from build123d import *

# Parameters (mm, degrees)
F3_DEPTH = 50
F2_R     = 25
F4_DEPTH = 15
F5_DEPTH = 35
F6_DEPTH = 35


with BuildPart() as f3:
    # F0 (on Front) → F3 (new body)
    with BuildSketch(Plane.XZ):
        with BuildLine():
            Line((0, 76), (-111, 76))
            ThreePointArc((-111, 76), (-187, 0), (-111, -76))
            Line((-111, -76), (0, -76))
            ThreePointArc((0, -76), (76, 0), (0, 76))
        make_face()
    extrude(amount=F3_DEPTH)

    # F2 (on offset) → F4 (cut)
    with BuildSketch(Plane.XZ.offset(19)):
        with Locations((-111, 0)):
            Circle(F2_R)
    extrude(amount=-F4_DEPTH, mode=Mode.SUBTRACT)

    # F2 (on offset) → F5 (cut)
    with BuildSketch(Plane.XZ.offset(19)):
        with Locations((-111, 0)):
            Circle(F2_R)
    extrude(amount=F5_DEPTH, mode=Mode.SUBTRACT)

    # F2 (on offset) → F6 (cut)
    with BuildSketch(Plane.XZ.offset(19)):
        with BuildLine():
            Line((0, 64), (-111, 64))
            ThreePointArc((-111, 64), (-175, 0), (-111, -64))
            Line((-111, -64), (0, -64))
            ThreePointArc((0, -64), (64, 0), (0, 64))
        make_face()
        with Locations((-111, 0)):
            Circle(F2_R, mode=Mode.SUBTRACT)
    extrude(amount=F6_DEPTH, mode=Mode.SUBTRACT)

    # F7 (on Right) → F8 (revolve, cut)
    with BuildSketch(Plane.YZ):
        Polygon((0, 11), (-2, 11), (-2, 18.5), (-7, 18.5), (-7, 23.5), (-19, 23.5), (-19, 0), (0, 0), align=None)
    revolve(axis=Axis((0, 0, 0), (0, 1, 0)), mode=Mode.SUBTRACT)


solid = f3.part
Build history of the part. All positions in model axes, mm. A direction names the side the tool comes from. Give positions to 0.01 mm unless a question says otherwise; leave off trailing zeros. Order: outer loops, then holes, each group sorted by start corner. A loop starts at its lowest first (then second) coordinate and runs counter-clockwise, first axis right, second up. Notation, with made-up numbers: M 70.25,12.25 L 79.25,12.25 A17 cw 79.25,19.25 Z; hole C 89,-23.5 d2. An arc over 180 degrees is marked long. Put each result on its own line as item: value.
Item 1: Cut at C-C on x = -36. Write the cut outline in (y, z), then the cut area to 3 significant figures.
Results are:
outline: M -50,-76 L 0,-76 L 0,76 L -50,76 L -50,64 L -19,64 L -19,-64 L -50,-64 Z
area: 3,630 mm2
Item 2: Cut at A-A on z = 0. Write the cut outline in (x, y).
Results are:
outline: M -187,-50 L -175,-50 L -175,-19 L -136,-19 L -136,-4 L -86,-4 L -86,-19 L -23.5,-19 L -23.5,-7 L -18.5,-7 L -18.5,-2 L -11,-2 L -11,0 L -187,0 Z; M 11,-2 L 18.5,-2 L 18.5,-7 L 23.5,-7 L 23.5,-19 L 64,-19 L 64,-50 L 76,-50 L 76,0 L 11,0 Z
Item 3: Cut at B-B on y = -45. Write the cut outline in (x, z), then the cut area to 3 significant figures.
Results are:
outline: M -111,-76 L 0,-76 A76 ccw 0,76 L -111,76 A76 ccw Z; hole M -111,-64 L 0,-64 A64 ccw 0,64 L -111,64 A64 ccw Z
area: 7,940 mm2
Item 4: Wall check: probe 1 along X at (y, z) = (-1.6, 0); probe 2 along Z at (x, y) = (-41, -28); probe 3 along Z at (x, y) = (-111, -9.5). Give the ranges that are in metal, low to high.
Results are:
probe 1: -187 to -11, 11 to 76
probe 2: -76 to -64, 64 to 76
probe 3: -76 to -25, 25 to 76
Item 5: Which spindle directions (+Z, -Z, +X, -X, +Y, -Y) get a long thin tool onto all of the face, cutting with end or side? Do faces 4 (the face through (-18.06, -4.54, -4.01)), 5 (the face through (-55, -25, 76)). Say none if no direction does.
Results are:
face 4: -Y
face 5: +Z, +X, -X, +Y, -Y
Item 6: Drop flat-ended pins along their axis: pin 1 Ø23.5 at (x, z) = (-3.5, -7) entering from -Y; pin 2 Ø5 at (y, z) = (-17.5, 10) entering from -X; pin 3 Ø25 at (x, z) = (-109, -1.5) entering from -Y. Give the stop position or say it passes through.
Results are:
pin 1: y = -7
pin 2: x = -186.63
pin 3: y = -4
Item 7: Pull direction X, two halves, no side cores. Call faces 1 (the face through (-186.98, -24.65, 1.67)), 2 (the face through (-10.74, -1.01, -2.38)), 3 (the face through (-56, -25, -76)): +X half, -X half, draft (parallel to the pull), parting line (faces both ways), or undercut.
Results are:
face 1: -X half
face 2: undercut
face 3: draft
Item 8: Cut at D-D on z = 28. Write the cut outline in (x, y), then the cut area to 3 significant figures.
Results are:
outline: M -181.65,-50 L -168.55,-50 L -168.55,-19 L 57.55,-19 L 57.55,-50 L 70.65,-50 L 70.65,0 L -181.65,0 Z
area: 5,610 mm2
